Part model, mm, in its own coordinate system. A direction names the side the tool comes from. Round coordinates to 2 decimals unless told otherwise and drop trailing zeros. Write each loop counter-clockwise with the first axis right and the second up, starting at its lowest first coordinate (ties: lowest second). Pieces come first, ordered by that corner, then holes. Notation, with made-up numbers: M 46.5,28.5 L 59.5,28.5 A35 cw 59.5,61.5 Z; hole C 73,26.5 d11. An arc over 180 degrees is marked long. Use a Markdown table: item, result. Add a question column.
1) Slice it at B-B on z = -0.5. Write the cut outline in (x, y).
2) Slice it at A-A on x = 4.5. Write the cut outline in (y, z), plus the area to 3 significant figures.
3) Which spindle directions (+Z, -Z, +X, -X, +Y, -Y) get a long thin tool onto all of the face, cutting with end or side? Do faces 4 (the face through (-4.7, -6.2, -1.6)), 5 (the face through (-1, 0, 0.8)), 6 (the face through (-3.9, -4.7, -1.6)). Say none if no direction does.
4) Slice it at C-C on z = 8. Write the cut outline in (x, y).
5) Wall check: probe 1 along X at (y, z) = (4.75, 0.25); probe 2 along X at (y, z) = (-3, 0.5); probe 3 along Z at (x, y) = (-2, 4.75). Give the ranges that are in metal, low to high.
6) Drop flat-ended pins along their axis: P1, Ø0.8, axis at y = -7, z = -0.5, coming from the -X side; P2, Ø5, axis at x = -18.5, y = 3, coming from the -Z side; P3, Ø0.6, axis at x = -4, z = -2, coming from the +Y side. Give the stop position or say it passes through.
7) Two-plate mould, pull along X, no slides. Class faces 1 (the face through (9.555, -2.868, 1.779)), 2 (the face through (-0.45, 4, -2)), 3 (the face through (10.2, -5.3, -0.5)): released by +X, released by -X, zero draft, split by the parting line, or undercut.
```python
from build123d import *

# Parameters (mm, degrees)
F0_W          = 20.4
F0_H          = 16.2
F1_DEPTH      = 1
F2_W          = 12
F2_H          = 4.5
F3_DEPTH      = 12
F3_DEPTH_BACK = 2
F4_W          = 4.7
F4_H          = 1
F5_DEPTH      = 2.6
F5_DEPTH_BACK = 3.8
F6_R          = 0.45
F7_DEPTH      = 3
F8_W          = 5.6
F8_H          = 5.6
F9_DEPTH      = 0.8
F10_W         = 4
F10_H         = 4
F11_DEPTH     = 0.8
F12_W         = 2
F12_H         = 1.25
F13_DEPTH     = 1.25
F14_W         = 1.25
F14_H         = 3
F15_DEPTH     = 1
F16_W         = 2
F16_H         = 1.25
F16_W_2       = 1.25
F16_H_2       = 2
F17_DEPTH     = 1.25
F18_W         = 1.6
F18_H         = 3
F19_DEPTH     = 1.15
F20_W         = 4.25
F20_H         = 3
F21_DEPTH     = 1.15
F22_W         = 14.25
F22_H         = 15
F23_DEPTH     = 8


with BuildPart() as f1:
    # F0 (on Top) → F1 (new body)
    with BuildSketch(Plane.XY):
        Rectangle(F0_W, F0_H)
    extrude(amount=-F1_DEPTH)

    # F2 (on face) → F3 (join, two sides)
    with BuildSketch(Plane(origin=(-10.2, 0, 0), x_dir=(0, -1, 0), z_dir=(-1, 0, 0))) as f3_sk:
        with Locations((0, 0.2)):
            Rectangle(F2_W, F2_H)
    extrude(amount=F3_DEPTH)
    extrude(f3_sk.sketch, amount=-F3_DEPTH_BACK)

    # F4 (on face) → F5 (join, two sides)
    with BuildSketch(Plane.YZ.offset(10.2)) as f5_sk:
        with Locations((0, -1.5)):
            Rectangle(F4_W, F4_H)
        with Locations((0, -0.5)):
            Rectangle(F4_W, F4_H)
        with BuildLine():
            Line((-3.375, 0), (-2.35, 0))
            Line((-2.35, 0), (2.35, 0))
            Line((2.35, 0), (3.375, 0))
            ThreePointArc((3.375, 0), (2.8817469144, 1.7567469144), (1.5461646096, 3))
            Line((1.5461646096, 3), (-1.5461646096, 3))
            ThreePointArc((-1.5461646096, 3), (-2.8817469144, 1.7567469144), (-3.375, 0))
        make_face()
    extrude(amount=F5_DEPTH)
    extrude(f5_sk.sketch, amount=-F5_DEPTH_BACK)

    # F6 (on face) → F7 (join)
    with BuildSketch(Plane(origin=(6.4, 0, 0), x_dir=(0, -1, 0), z_dir=(-1, 0, 0))):
        with Locations((0, 0.5)):
            Circle(F6_R)
    extrude(amount=F7_DEPTH)

    # F8 (on face) → F9 (join)
    with BuildSketch(Plane.XY):
        with Locations((-6.3, -0.75)):
            Rectangle(F8_W, F8_H)
    extrude(amount=F9_DEPTH)

    # F10 (on face) → F11 (join)
    with BuildSketch(Plane.XY):
        with Locations((2.15, -4.1)):
            Rectangle(F10_W, F10_H)
    extrude(amount=F11_DEPTH)

    # F12 (on face) → F13 (join)
    with BuildSketch(Plane.XY):
        with Locations((-5.4, 4.975)):
            Rectangle(F12_W, F12_H)
    extrude(amount=F13_DEPTH)

    # F14 (on face) → F15 (join)
    with BuildSketch(Plane.XY):
        with Locations((6.775, 6.1)):
            Rectangle(F14_W, F14_H)
    extrude(amount=F15_DEPTH)

    # F16 (on face) → F17 (join)
    with BuildSketch(Plane(origin=(0, 0, -1), x_dir=(1, 0, 0), z_dir=(0, 0, -1))):
        with Locations((0.55, -4.475)):
            Rectangle(F16_W, F16_H)
        with Locations((-3.275, -1.1)):
            Rectangle(F16_W_2, F16_H_2)
        with Locations((-0.775, 6.1)):
            Rectangle(F16_W_2, F16_H_2)
    extrude(amount=F17_DEPTH)

    # F18 (on face) → F19 (join)
    with BuildSketch(Plane(origin=(0, 0, -1), x_dir=(1, 0, 0), z_dir=(0, 0, -1))):
        with Locations((-4.15, -5.7)):
            Rectangle(F18_W, F18_H)
        with Locations((-3.9, 6.2)):
            Rectangle(F18_W, F18_H)
    extrude(amount=F19_DEPTH)

    # F20 (on face) → F21 (join)
    with BuildSketch(Plane(origin=(0, 0, -1), x_dir=(1, 0, 0), z_dir=(0, 0, -1))):
        with Locations((6.175, -4.27)):
            Rectangle(F20_W, F20_H)
    extrude(amount=F21_DEPTH)

    # F22 (on face) → F23 (join)
    with BuildSketch(Plane.XY.offset(0.8)):
        with Locations((-0.725, 0)):
            Rectangle(F22_W, F22_H)
    extrude(amount=F23_DEPTH)


solid = f1.part
```
Entries:
| question | item | result |
|---|---|---|
| 1 | outline | M -22.2,-6 L -10.2,-6 L -10.2,-8.1 L 10.2,-8.1 L 10.2,-2.35 L 12.8,-2.35 L 12.8,2.35 L 10.2,2.35 L 10.2,8.1 L -10.2,8.1 L -10.2,6 L -22.2,6 Z |
| 2 | outline | M -8.1,-1 L 2.77,-1 L 2.77,-2.15 L 5.77,-2.15 L 5.77,-1 L 8.1,-1 L 8.1,0 L -8.1,0 Z; M -7.5,0.8 L -0.34,0.8 A0.45 ccw long 0.34,0.8 L 7.5,0.8 L 7.5,8.8 L -7.5,8.8 Z |
| 2 | area | 140 mm^2 |
| 3 | face 4 | -Z, -Y |
| 3 | face 5 | none |
| 3 | face 6 | -Z, +X |
| 4 | outline | M -7.85,-7.5 L 6.4,-7.5 L 6.4,7.5 L -7.85,7.5 Z |
| 5 | probe 1 | x = -22.2 to -8.2, -6.4 to -4.4, 6.15 to 7.4 |
| 5 | probe 2 | x = -22.2 to -3.5, 0.15 to 4.15, 6.4 to 12.8 |
| 5 | probe 3 | z = -1 to 0, 0.8 to 8.8 |
| 6 | P1 | stops at x = -10.2 |
| 6 | P2 | stops at z = -2.05 |
| 6 | P3 | stops at y = 7.2 |
| 7 | face 1 | zero draft |
| 7 | face 2 | undercut |
| 7 | face 3 | released by +X |
